CAD build for the part. Positions are in the model's coordinates, mm. A direction names the side the tool comes from. Give positions to 0.01 mm unless a question says otherwise; leave off trailing zeros. Loops run counter-clockwise (first coordinate to the right, second up) from the corner with the lowest first, then second, coordinate; pieces in that order, holes last.
```python
from build123d import *

# Parameters (mm, degrees)
SKETCH_2_R          = 6.05
SKETCH_2_R_2        = 2.05
EXTRUDE_1_DEPTH     = 5
EXTRUDE_1_2_DEPTH   = 5
EXTRUDE_1_3_DEPTH   = 5
EXTRUDE_1_4_DEPTH   = 5
SKETCH_6_R          = 2.05
EXTRUDE_1_5_DEPTH   = 5
SKETCH_11_R         = 3.25
SKETCH_11_W         = 19
SKETCH_11_H         = 11.05
SKETCH_11_W_2       = 20
SKETCH_11_H_2       = 17
SKETCH_11_W_3       = 9
SKETCH_11_H_3       = 12.5
SKETCH_11_W_4       = 11.5
SKETCH_11_H_4       = 5
CUT_EXTRUDE_4_DEPTH = 151.533194014
CUT_EXTRUDE_5_DEPTH = 153.920706577


with BuildPart() as part:
    # 草图2 → Extrude 1 (new body)
    with BuildSketch(Plane(origin=(0, 0, 0), x_dir=(-1, 0, 0), z_dir=(0, -1, 0))):
        with Locations((-103.2, -9.35)):
            Circle(SKETCH_2_R)
        with Locations((-103.2, -9.35)):
            Circle(SKETCH_2_R_2, mode=Mode.SUBTRACT)
    extrude(amount=EXTRUDE_1_DEPTH)



with BuildPart() as body_2:
    # 草图2 → Extrude 1 2 (new body)
    with BuildSketch(Plane(origin=(0, 0, 0), x_dir=(-1, 0, 0), z_dir=(0, -1, 0))):
        with Locations((-63.2, -9.35)):
            Circle(SKETCH_2_R)
        with Locations((-63.2, -9.35)):
            Circle(SKETCH_2_R_2, mode=Mode.SUBTRACT)
    extrude(amount=EXTRUDE_1_2_DEPTH)


with BuildPart() as body_3:
    # 草图2 → Extrude 1 3 (new body)
    with BuildSketch(Plane(origin=(0, 0, 0), x_dir=(-1, 0, 0), z_dir=(0, -1, 0))):
        with Locations((-63.2, -64.25)):
            Circle(SKETCH_2_R)
        with Locations((-63.2, -64.25)):
            Circle(SKETCH_2_R_2, mode=Mode.SUBTRACT)
    extrude(amount=EXTRUDE_1_3_DEPTH)


with BuildPart() as body_4:
    # 草图2 → Extrude 1 4 (new body)
    with BuildSketch(Plane(origin=(0, 0, 0), x_dir=(-1, 0, 0), z_dir=(0, -1, 0))):
        with Locations((-103.2, -64.25)):
            Circle(SKETCH_2_R)
        with Locations((-103.2, -64.25)):
            Circle(SKETCH_2_R_2, mode=Mode.SUBTRACT)
    extrude(amount=EXTRUDE_1_4_DEPTH)


with BuildPart() as part_1:
    add(part.part)

    add(body_2.part)  # Extrude 1 5 merges body 2

    add(body_3.part)  # Extrude 1 5 merges body 3

    add(body_4.part)  # Extrude 1 5 merges body 4
    # 草图6 → Extrude 1 5 (add)
    with BuildSketch(Plane(origin=(0, 0, 0), x_dir=(1, 0, 0), z_dir=(0, 1, 0))):
        with BuildLine():
            Line((127.2, 1.45), (109.046152581, 1.45))
            ThreePointArc((109.046152581, 1.45), (107.496959242, 1.246550698), (106.052826672, 0.65))
            Line((106.052826672, 0.65), (63.2, 0.65))
            Line((63.2, 0.65), (45.7, 0.65))
            ThreePointArc((45.7, 0.65), (43.932233047, -0.082233047), (43.2, -1.85))
            Line((43.2, -1.85), (43.2, -64.3))
            ThreePointArc((43.2, -64.3), (44.957359313, -68.542640687), (49.2, -70.3))
            Line((49.2, -70.3), (103.2, -70.3))
            ThreePointArc((103.2, -70.3), (105.311182702, -73.645742753), (109.046152581, -74.95))
            Line((109.046152581, -74.95), (127.2, -74.95))
            ThreePointArc((127.2, -74.95), (131.442640687, -73.192640687), (133.2, -68.95))
            Line((133.2, -68.95), (133.2, -4.55))
            ThreePointArc((133.2, -4.55), (131.442640687, -0.307359313), (127.2, 1.45))
        make_face()
        with Locations(Location((103.2, -9.35, 0), (0, 0, 270))):
            Circle(SKETCH_6_R, mode=Mode.SUBTRACT)
        with Locations(Location((103.2, -64.25, 0), (0, 0, 270))):
            Circle(SKETCH_6_R, mode=Mode.SUBTRACT)
        with Locations(Location((63.2, -64.25, 0), (0, 0, 270))):
            Circle(SKETCH_6_R, mode=Mode.SUBTRACT)
        with Locations(Location((63.2, -9.35, 0), (0, 0, 90))):
            Circle(SKETCH_6_R, mode=Mode.SUBTRACT)
    extrude(amount=-EXTRUDE_1_5_DEPTH)

    # 草图11 → 切除-拉伸4 (cut, through all)
    with BuildSketch(Plane(origin=(0, -5, 5), x_dir=(1, 0, 0), z_dir=(0, -1, 0))):
        Polygon((49.2, 13.05), (43.2, 13.05), (43.2, 6.35), (45.8, 6.35), (45.8, -3.15), (58.8, -3.15), (58.8, 8.85), (49.2, 8.85), align=None)
        with Locations(Location((57.9, 37.35, 0), (0, 0, 90))):
            Circle(SKETCH_11_R)
        with Locations((82.7, 59.775)):
            Rectangle(SKETCH_11_W, SKETCH_11_H)
        with Locations((117.7, 4.85)):
            Rectangle(SKETCH_11_W_2, SKETCH_11_H_2)
        with Locations((94, 24.1)):
            Rectangle(SKETCH_11_W_3, SKETCH_11_H_3)
        with Locations((114.45, 61.35)):
            Rectangle(SKETCH_11_W_4, SKETCH_11_H_4)
        with BuildLine():
            ThreePointArc((106.2, 29.9), (102.95, 26.65), (106.2, 23.4))
            Line((106.2, 23.4), (108.2, 23.4))
            Line((108.2, 23.4), (108.2, 15.85))
            Line((108.2, 15.85), (125.2, 15.85))
            Line((125.2, 15.85), (125.2, 25.85))
            Line((125.2, 25.85), (124.2, 25.85))
            Line((124.2, 25.85), (124.2, 57.35))
            Line((124.2, 57.35), (109.7, 57.35))
            Line((109.7, 57.35), (109.7, 56))
            Line((109.7, 56), (106.2, 56))
            ThreePointArc((106.2, 56), (102.95, 52.75), (106.2, 49.5))
            Line((106.2, 49.5), (109.7, 49.5))
            Line((109.7, 49.5), (109.7, 47.3))
            Line((109.7, 47.3), (106.2, 47.3))
            ThreePointArc((106.2, 47.3), (102.95, 44.05), (106.2, 40.8))
            Line((106.2, 40.8), (109.7, 40.8))
            Line((109.7, 40.8), (109.7, 38.6))
            Line((109.7, 38.6), (106.2, 38.6))
            ThreePointArc((106.2, 38.6), (102.95, 35.35), (106.2, 32.1))
            Line((106.2, 32.1), (109.7, 32.1))
            Line((109.7, 32.1), (109.7, 29.9))
            Line((109.7, 29.9), (106.2, 29.9))
        make_face()
    extrude(amount=-CUT_EXTRUDE_4_DEPTH, mode=Mode.SUBTRACT)

    # 草图12 → Cut-Extrude 5 (cut, through all)
    with BuildSketch(Plane.XZ.offset(5)):
        with BuildLine():
            Line((58.8, -0.65), (58.8, 1.85))
            Line((58.8, 1.85), (45.8, 1.85))
            Line((45.8, 1.85), (45.8, 11.35))
            Line((45.8, 11.35), (43.2, 11.35))
            Line((43.2, 11.35), (43.2, 1.85))
            ThreePointArc((43.2, 1.85), (43.932233047, 0.082233047), (45.7, -0.65))
            Line((45.7, -0.65), (58.8, -0.65))
        make_face()
    extrude(amount=-CUT_EXTRUDE_5_DEPTH, mode=Mode.SUBTRACT)


solid = part_1.part
```
1. Drop flat-ended pins along their axis: pin 1 (2 mm diameter, centred on x = 61, y = -1.5, fed in from +Z); pin 2 (6 mm diameter, centred on x = 57.9, z = 42.35, fed in from +Y); pin 3 (1 mm diameter, centred on x = 108.5, y = -2, fed in from -Z); pin 4 (2.5 mm diameter, centred on x = 46, y = -3, fed in from -Z). Give the stop position or say it passes through.
Responses:
pin 1: stops at z = 70.3
pin 2: passes through
pin 3: stops at z = -1.45
pin 4: stops at z = 18.05
2. Saw through at B-B, the plane z = 9.35. List the corners of the cut face in (x, y), and give its area (3 significant figures).
Responses:
outline: (58.8, -5) - (61.15, -5) - (61.15, 0) - (58.8, 0) - close; (65.25, -5) - (101.15, -5) - (101.15, 0) - (65.25, 0) - close; (105.25, -5) - (107.7, -5) - (107.7, 0) - (105.25, 0) - close; (127.7, -5) - (133.2, -5) - (133.2, 0) - (127.7, 0) - close
area: 231 mm2
3. Saw through at C-C, the plane x = 56. List the corners of the cut face in (y, z).
Responses:
outline: (-5, 13.85) - (0, 13.85) - (0, 39.71) - (-5, 39.71) - close; (-5, 44.99) - (0, 44.99) - (0, 70.3) - (-5, 70.3) - close
4. Tool access for faces 1 (the face through (94, -3, 22.85)), 2 (the face through (54, -3, 13.85)), 3 (the face through (92.2, -3, 65)), 4 (the face through (61, -2, 70.3)), 5 (the face through (133.2, -2, 37)): list every direction of +Z, -Z, +X, -X, +Y, -Y with a clear straight run to the whole face (end or side of a thin tool).
Responses:
face 1: +Y, -Y
face 2: -Z, -X, +Y, -Y
face 3: +Z, +Y, -Y
face 4: +Z, -X, +Y, -Y
face 5: +Z, -Z, +X, +Y, -Y
5. Probe line 1 along Z through (x, y) = (113, -1.2); line 2 along X through (y, z) = (-2.15, 64.25); line 3 along Z through (x, y) = (63, -1.6). List the from-to ranges inside material, lowest first.
Responses:
line 1: z = -1.45 to 1.35, 18.35 to 20.85, 62.35 to 63.85, 68.85 to 74.95
line 2: x = 43.2 to 61.15, 65.25 to 73.2, 92.2 to 101.15, 105.25 to 108.7, 120.2 to 133.2
line 3: z = -0.65 to 7.31, 11.39 to 62.21, 66.29 to 70.3
6. Saw through at D-D, the plane z = 42. List the corners of the cut face in (x, y), and give its area (3 significant figures).
Responses:
outline: (43.2, -5) - (54.67, -5) - (54.67, 0) - (43.2, 0) - close; (61.13, -5) - (103.4, -5) - (103.4, 0) - (61.13, 0) - close; (124.2, -5) - (133.2, -5) - (133.2, 0) - (124.2, 0) - close
area: 314 mm2
7. Saw through at A-A, the plane z = 57.75. List the corners of the cut face in (x, y), and give its area (3 significant figures).
Responses:
outline: (43.2, -5) - (102.95, -5) - (102.95, 0) - (43.2, 0) - close; (124.2, -5) - (133.2, -5) - (133.2, 0) - (124.2, 0) - close
area: 344 mm2
